Verification items for the finished model (mm, model axes). A direction names the side the tool comes from. Coordinates: 2 decimals unless noted, no trailing zeros. Write each loop counter-clockwise with the first axis right and the second up, starting at its lowest first coordinate (ties: lowest second). Pieces come first, ordered by that corner, then holes. Notation, with made-up numbers: (54.25, 75) -> (91.25, 75) arc R19 cw to (91.25, 85) -> close; hole circle Ø4 at (-17, 39.25). An arc over 180 degrees is marked (long way). Answer in a Markdown table with one row per item.
```python
from build123d import *

# Parameters (mm, degrees)
CROQUIS1_W            = 5
CROQUIS1_H            = 7.5
CROQUIS2_R            = 0.5
CROQUIS2_W            = 4
CROQUIS2_H            = 1
CROQUIS2_H_2          = 2
CORTAR_EXTRUIR1_DEPTH = 8.5
CROQUIS3_W            = 8
CROQUIS3_H            = 3.5
CORTAR_EXTRUIR2_DEPTH = 3.5


with BuildPart() as part:
    # Croquis1 → Revolución1 (revolve)
    with BuildSketch(Plane.XY):
        with Locations((2.5, 3.75)):
            Rectangle(CROQUIS1_W, CROQUIS1_H)
    revolve(axis=Axis((0, 0, 0), (0, 1, 0)))

    # Croquis2 → Cortar-Extruir1 (cut, through all)
    with BuildSketch(Plane(origin=(0, 7.5, 0), x_dir=(1, 0, 0), z_dir=(0, 1, 0))):
        with Locations((-3, 0)):
            Circle(CROQUIS2_R)
        with BuildLine():
            Line((-2, 0.5), (-3, 0.5))
            ThreePointArc((-3, 0.5), (-2.646446609, 0.353553391), (-2.5, 0))
            ThreePointArc((-2.5, 0), (-2.646446609, -0.353553391), (-3, -0.5))
            Line((-3, -0.5), (-2, -0.5))
            Line((-2, -0.5), (-2, 0.5))
        make_face()
        Rectangle(CROQUIS2_W, CROQUIS2_H)
        with Locations((0, 1.5)):
            Rectangle(CROQUIS2_W, CROQUIS2_H_2)
        with Locations((0, -1.5)):
            Rectangle(CROQUIS2_W, CROQUIS2_H_2)
        with BuildLine():
            Line((3, 0.5), (2, 0.5))
            Line((2, 0.5), (2, -0.5))
            Line((2, -0.5), (3, -0.5))
            ThreePointArc((3, -0.5), (2.5, 0), (3, 0.5))
        make_face()
        with Locations((3, 0)):
            Circle(CROQUIS2_R)
    extrude(amount=-CORTAR_EXTRUIR1_DEPTH, mode=Mode.SUBTRACT)

    # Croquis3 → Cortar-Extruir2 (cut)
    with BuildSketch(Plane(origin=(0, 7.5, 0), x_dir=(1, 0, 0), z_dir=(0, 1, 0))):
        Rectangle(CROQUIS3_W, CROQUIS3_H)
    extrude(amount=-CORTAR_EXTRUIR2_DEPTH, mode=Mode.SUBTRACT)


solid = part.part
```
1. Tool access check on faces 5 (the flat face through (3, 6, -1.75)), 6 (the cylindrical face through (3.5, 2, 0)). Record the directions out of +Z, -Z, +X, -X, +Y, -Y that give a thin tool (end or side, any length) a straight path to the whole face; none if there is none.
Geometry says:
| item | result |
|---|---|
| face 5 | +Y |
| face 6 | +Y, -Y |
2. Depth check by flat-ended pin: P1, Ø1.6, axis at x = 3, z = -0.5, coming from the +Y side; P2, Ø1, axis at y = 5, z = 2, coming from the -X side; P3, Ø1.1, axis at x = 2.5, y = 2, coming from the -Z side. Enter the tip coordinate at first touch or a pass-through.
Geometry says:
| item | result |
|---|---|
| P1 | y = 4 |
| P2 | x = -4.77 |
| P3 | z = -4.6 |
3. Section check D-D, the plane y = 4.75. Record the boundary of the cut face in (x, z).
Geometry says:
| item | result |
|---|---|
| outline | circle Ø10 at (0, 0); hole (-4, -1.75) -> (-2, -1.75) -> (-2, -2.5) -> (2, -2.5) -> (2, -1.75) -> (4, -1.75) -> (4, 1.75) -> (2, 1.75) -> (2, 2.5) -> (-2, 2.5) -> (-2, 1.75) -> (-4, 1.75) -> close |
4. Section check C-C, the plane z = 0. Record the boundary of the cut face in (x, y), plus the area to 3 significant figures.
Geometry says:
| item | result |
|---|---|
| outline | (-5, 0) -> (-3.5, 0) -> (-3.5, 4) -> (-4, 4) -> (-4, 7.5) -> (-5, 7.5) -> close; (3.5, 0) -> (5, 0) -> (5, 7.5) -> (4, 7.5) -> (4, 4) -> (3.5, 4) -> close |
| area | 19.0 mm^2 |
5. Thickness scan on line 1 (Z direction, x = 0, y = 6.75); line 2 (Z direction, x = 3, y = 6.25); line 3 (Z direction, x = -4, y = 2.25). Record the ranges inside material, lowest first. Write a range as from..to.
Geometry says:
| item | result |
|---|---|
| line 1 | -5..-2.5, 2.5..5 |
| line 2 | -4..-1.75, 1.75..4 |
| line 3 | -3..3 |
6. Section check A-A, the plane x = 0. Record the boundary of the cut face in (y, z).
Geometry says:
| item | result |
|---|---|
| outline | (0, -5) -> (7.5, -5) -> (7.5, -2.5) -> (0, -2.5) -> close; (0, 2.5) -> (7.5, 2.5) -> (7.5, 5) -> (0, 5) -> close |
7. Mould release check, pull along X, two halves, no side actions. Record for faces 1 (the flat face through (-2.2, 0, 1)), 2 (the flat face through (0, 4, -2.5)), 3 (the cylindrical face through (-1.08, 3.8, 4.88)), 4 (the flat face through (-3, 6, -1.75)): released by +X, released by -X, zero draft, split by the parting line, or undercut.
Geometry says:
| item | result |
|---|---|
| face 1 | zero draft |
| face 2 | undercut |
| face 3 | split by the parting line |
| face 4 | undercut |
8. Section check B-B, the plane y = 1.5. Record the boundary of the cut face in (x, z).
Geometry says:
| item | result |
|---|---|
| outline | circle Ø10 at (0, 0); hole (-3, -0.5) -> (-2, -0.5) -> (-2, -2.5) -> (2, -2.5) -> (2, -0.5) -> (3, -0.5) arc R0.5 ccw to (3, 0.5) -> (2, 0.5) -> (2, 2.5) -> (-2, 2.5) -> (-2, 0.5) -> (-3, 0.5) arc R0.5 ccw to start |
